```python
from build123d import *

# Parameters (mm, degrees)
F0_R     = 12.05
F1_DEPTH = 20
F2_R     = 5
F3_R     = 200
F4_DEPTH = 5


with BuildPart() as f1:
    # F0 (on Top) → F1 (new body)
    with BuildSketch(Plane.XY):
        Polygon((750, 0), (0, 0), (0, -750), (50, -750), (750, -50), align=None)
        with Locations((250, -250)):
            Circle(F0_R, mode=Mode.SUBTRACT)
    extrude(amount=F1_DEPTH)

    # F2
    f2_edges = [f1.edges().sort_by_distance(p)[0] for p in [
        (0, -750, 10),
        (750, 0, 10),
        (0, 0, 10),
    ]]
    fillet(f2_edges, radius=F2_R)

    # F3 (on Top) → F4 (cut)
    with BuildSketch(Plane.XY):
        with Locations((250, -250)):
            Circle(F3_R)
    extrude(amount=F4_DEPTH, mode=Mode.SUBTRACT)


solid = f1.part
```
Geometry check sheet. Reference: the model listing, model coordinates, mm. A direction names the side the tool comes from. Round coordinates to 2 decimals unless told otherwise and drop trailing zeros. Loops run counter-clockwise (first coordinate to the right, second up) from the corner with the lowest first, then second, coordinate; pieces in that order, holes last. Notation, with made-up numbers: (72, -11.5) - (86, -11.5) arc R9 ccw to (86, -1.5) - close; hole circle Ø3 at (4, -26). An arc over 180 degrees is marked (long way). Write each question's results on one line, items separated by ' | '. Start each with the question number.
Q1. Cross-section at A-A on y = -250. Enter the section's corners in (x, z), and give its area (3 significant figures).
Q2. Cross-section at D-D on y = -499.5. Enter the section's corners in (x, z).
Q3. Cross-section at B-B on x = 250. Enter the section's corners in (y, z), and give its area (3 significant figures).
Q4. Gauge pin test, flat ends, axial feed: P1, Ø12, axis at y = -448.5, z = 12.5, coming from the +X side; P2, Ø6, axis at x = 243.5, z = 8.5, coming from the -Y side. Record the tip position at first contact, or that the pin passes through.
Q5. Cross-section at C-C on z = 10. Enter the section's corners in (x, y), and give its area (3 significant figures).
Q6. Thickness scan on line 1 (Y direction, x = 250, z = 11.5); line 2 (Z direction, x = 111.5, y = -326); line 3 (X direction, y = -250, z = 9.25). Record the ranges inside material, lowest first. Write a range as [from, to].
Q7. Access from +Z, -Z, +X, -X, +Y, -Y to the whole of each face (thin tool, end or side, straight path). Record for faces 5 (the flat face through (247, -292, 5)), 6 (the flat face through (395, -405, 10)).
Q8. Release check for a two-part mould opening along X. For faces 1 (the flat face through (27, -750, 10)), 2 (the flat face through (0, -370, 10)), 3 (the flat face through (750, -28, 10)), 4 (the cylindrical face through (261.13, -254.62, 12.4)) record: +X half, -X half, draft (parallel to the pull), parting line (faces both ways), or undercut.
Answers below:
1) outline: (0, 0) - (50, 0) - (50, 5) - (237.95, 5) - (237.95, 20) - (0, 20) - close; (262.05, 5) - (450, 5) - (450, 0) - (550, 0) - (550, 20) - (262.05, 20) - close | area: 8,640 mm²
2) outline: (0, 0) - (300.5, 0) - (300.5, 20) - (0, 20) - close
3) outline: (-550, 0) - (-450, 0) - (-450, 5) - (-262.05, 5) - (-262.05, 20) - (-550, 20) - close; (-237.95, 5) - (-50, 5) - (-50, 0) - (0, 0) - (0, 20) - (-237.95, 20) - close | area: 8,640 mm²
4) P1: stops at x = 357.5 | P2: stops at y = -559.5
5) outline: (0, -745) arc R5 ccw to (5, -750) - (50, -750) - (750, -50) - (750, -5) arc R5 ccw to (745, 0) - (5, 0) arc R5 ccw to (0, -5) - close; hole circle Ø24.1 at (250, -250) | area: 317,000 mm²
6) line 1: y = [-550, -262.05], [-237.95, 0] | line 2: z = [5, 20] | line 3: x = [0, 237.95], [262.05, 550]
7) face 5: -Z | face 6: +Z, -Z, +X, -Y
8) face 1: draft | face 2: -X half | face 3: +X half | face 4: undercut
